For this review, take the finished solid that the model builds, in its own axes (mm). Face numbers are marked on the shaded views. A direction names the side the tool comes from. Round coordinates to 2 decimals unless told otherwise and drop trailing zeros. Order: outer loops, then holes, each group sorted by start corner. A loop starts at its lowest first (then second) coordinate and runs counter-clockwise, first axis right, second up. Notation, with made-up numbers: M 75,86 L 99,86 A15 ccw 99,114 Z; hole C 28,52 d10. An arc over 180 degrees is marked long. Put each result on its own line as item: value.
from build123d import *

# Parameters (mm, degrees)
SKETCH1_W           = 17.5
SKETCH1_H           = 11
BOSS_EXTRUDE1_DEPTH = 2
SKETCH2_W           = 17.5
SKETCH2_H           = 2
BOSS_EXTRUDE2_DEPTH = 64
SKETCH3_W           = 17.5
SKETCH3_H           = 11
BOSS_EXTRUDE3_DEPTH = 2
SKETCH4_R           = 1.25
CUT_EXTRUDE1_DEPTH  = 68


with BuildPart() as part:
    # Sketch1 → Boss-Extrude1 (new body)
    with BuildSketch(Plane(origin=(0, 0, 0), x_dir=(0, 0, -1), z_dir=(1, 0, 0))):
        with Locations((-48.014351082, 3.54)):
            Rectangle(SKETCH1_W, SKETCH1_H)
    extrude(amount=BOSS_EXTRUDE1_DEPTH)

    # Sketch2 → Boss-Extrude2 (add)
    with BuildSketch(Plane(origin=(2, 0, 0), x_dir=(0, 0, -1), z_dir=(1, 0, 0))):
        with Locations((-48.014351082, -0.96)):
            Rectangle(SKETCH2_W, SKETCH2_H)
    extrude(amount=BOSS_EXTRUDE2_DEPTH)

    # Sketch3 → Boss-Extrude3 (add)
    with BuildSketch(Plane(origin=(66, 0, 0), x_dir=(0, 0, -1), z_dir=(1, 0, 0))):
        with Locations((-48.014351082, 3.54)):
            Rectangle(SKETCH3_W, SKETCH3_H)
    extrude(amount=BOSS_EXTRUDE3_DEPTH)

    # Sketch4 → Cut-Extrude1 (cut)
    with BuildSketch(Plane(origin=(68, 0, 0), x_dir=(0, 0, -1), z_dir=(1, 0, 0))):
        with Locations((-52.014351082, 6.04)):
            Circle(SKETCH4_R)
        with Locations((-44.014351082, 6.04)):
            Circle(SKETCH4_R)
    extrude(amount=-CUT_EXTRUDE1_DEPTH, mode=Mode.SUBTRACT)


solid = part.part
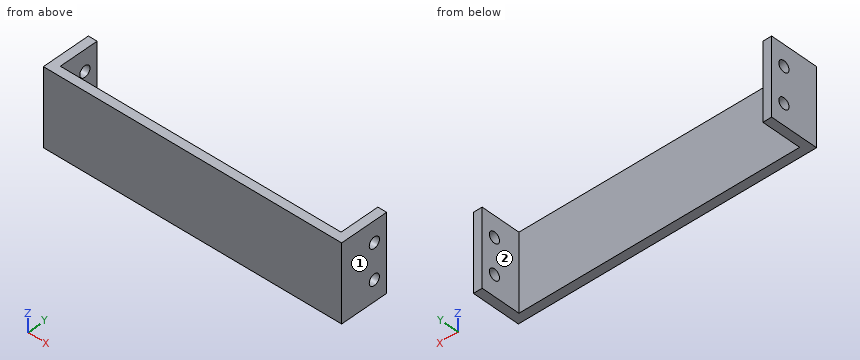
(1) Add section B-B on z = 54.25. Give the boundary of the cut face in (x, y), then the cut area to 3 significant figures.
A:
outline: M 0,-1.96 L 68,-1.96 L 68,9.04 L 66,9.04 L 66,0.04 L 2,0.04 L 2,9.04 L 0,9.04 Z
area: 172 mm2
(2) Add section A-A on y = 8. Give the boundary of the cut face in (x, z), then the cut area to 3 significant figures.
A:
outline: M 0,39.26 L 2,39.26 L 2,56.76 L 0,56.76 Z; M 66,39.26 L 68,39.26 L 68,56.76 L 66,56.76 Z
area: 70.0 mm2
(3) For the marked faces 1 and 2, list the 3-axis set-ups (+Z, -Z, +X, -X, +Y, -Y) from which the entire face can be reached by the end or side of a thin tool; tool diameter is ignored.
A:
face 1: +Z, -Z, +X, +Y, -Y
face 2: +Z, -Z, +Y
(4) To check wall thickness, follow L1, parallel to X at y = 4.75, z = 48.5; L2, parallel to Y at x = 22, z = 49.75. State the ranges of each line that lie inside material, in increasing order.
A:
L1: x = 0 to 2, 66 to 68
L2: y = -1.96 to 0.04
(5) Add section C-C on x = 19. Give the boundary of the cut face in (y, z), then the cut area to 3 significant figures.
A:
outline: M -1.96,39.26 L 0.04,39.26 L 0.04,56.76 L -1.96,56.76 Z
area: 35.0 mm2
(6) Insertion check: pin 1 Ø5 at (x, y) = (53, 3.5) entering from +Z. The pin has a flat end and moves straight along its axis. Give the tip position at first contact, or say it passes through.
A:
pin 1: passes through
